Autodesk Fusion 360 part; units mm, degrees
sketch "Sketch1" plane through (0, 0, 0) normal (1, 0, 0) x (0, 0, -1)
  line L0 (-10, 140) -> (10, 140)
  line L1 (10, 140) -> (10, -140)
  line L2 (10, -140) -> (-10, -140)
  line L3 (-10, -140) -> (-10, 140)
  circle A0 centre (0, 130) radius 3
  dimension "d1" = 20
  dimension "d2" = 280
  dimension "d3" = 6
  dimension "d4" = 10
extrude "Extrude1" add sketch "Sketch1" along normal blind 6
Read the model definition and answer for the solid it produces. Units are mm, in the model's axes. Give positions to 0.01 mm unless a question says otherwise; leave off trailing zeros. Write each loop counter-clockwise with the first axis right and the second up, starting at its lowest first coordinate (ties: lowest second). Pieces come first, ordered by that corner, then holes. Notation, with made-up numbers: (87.25, 20.5) - (136.25, 20.5) arc R10 cw to (136.25, 35.5) - close; hole circle Ø6 at (0, 6.25). An arc over 180 degrees is marked (long way). Use CSV: the item, a comma, the result in double quotes. Start each with the question number.
(1) Find section A-A (z = 0). Give the vertices of the cut face in (x, y).
(2) Find section B-B (y = 130). Give the vertices of the cut face in (x, z).
(3) Consider line 1 along Y through (x, z) = (1.9, 0); line 2 along Z through (x, y) = (1.9, 130); line 3 along Y through (x, z) = (2.25, 2.75). Determine where each line is inside the solid, lowest interval first.
(4) Given P1, Ø8, axis at y = 130, z = 0, coming from the -X side, flat-ended and moving along its own axis, determine where the tip first touches the part or whether it passes through.
Findings below:
1,outline,"(0, -140) - (6, -140) - (6, 127) - (0, 127) - close; (0, 133) - (6, 133) - (6, 140) - (0, 140) - close"
2,outline,"(0, -10) - (6, -10) - (6, -3) - (0, -3) - close; (0, 3) - (6, 3) - (6, 10) - (0, 10) - close"
3,line 1,"-140 to 127, 133 to 140"
3,line 2,"-10 to -3, 3 to 10"
3,line 3,"-140 to 128.8, 131.2 to 140"
4,P1,"x = 0"
